For this review, use the dimensioned drawing (mm, ordinates from the lowest corner) and the shaded views. Coordinates: 2 decimals unless noted, no trailing zeros. Write each loop counter-clockwise with the first axis right and the second up, starting at its lowest first coordinate (ties: lowest second). Pieces come first, ordered by that corner, then holes. Notation, with made-up numbers: (86.25, 60.5) - (117.25, 60.5) arc R27 cw to (117.25, 97.5) - close; hole circle Ø4 at (6, 33). An arc over 180 degrees is marked (long way). Put each result on its own line as item: value.
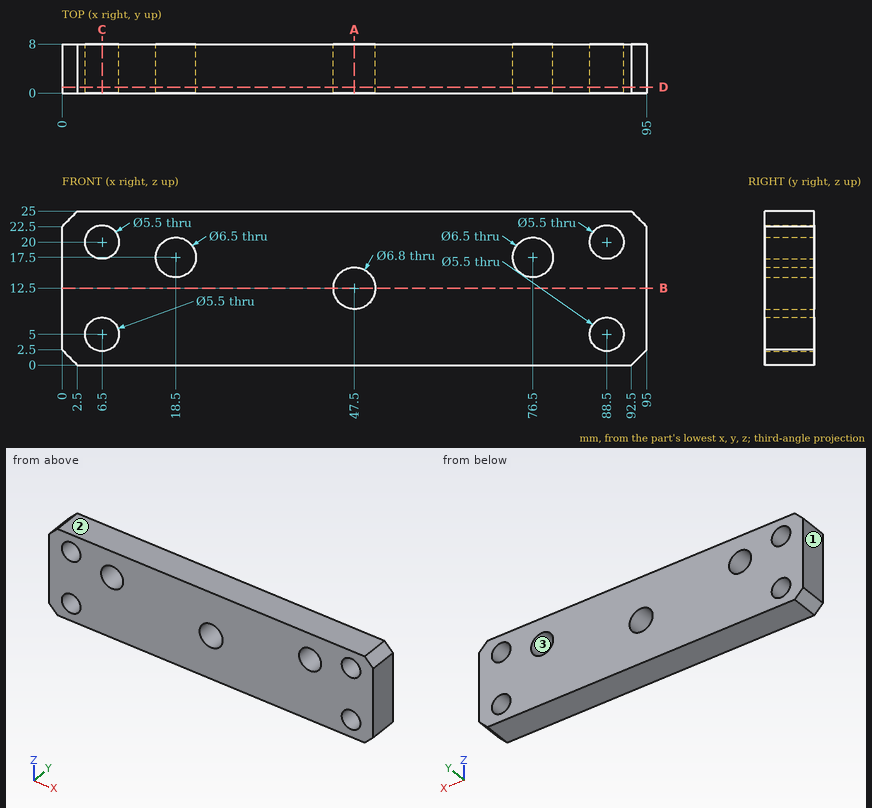
1. Consider section B-B on z = 12.5. State the section outline as (x, y) points, plus the area to 3 significant figures.
Determined:
outline: (0, 0) - (44.1, 0) - (44.1, 8) - (0, 8) - close; (50.9, 0) - (95, 0) - (95, 8) - (50.9, 8) - close
area: 706 mm^2
2. Consider section A-A on x = 47.5. State the section outline as (y, z) points, plus the area to 3 significant figures.
Determined:
outline: (0, 0) - (8, 0) - (8, 9.1) - (0, 9.1) - close; (0, 15.9) - (8, 15.9) - (8, 25) - (0, 25) - close
area: 146 mm^2
3. Consider section C-C on x = 6.5. State the section outline as (y, z) points.
Determined:
outline: (0, 0) - (8, 0) - (8, 2.25) - (0, 2.25) - close; (0, 7.75) - (8, 7.75) - (8, 17.25) - (0, 17.25) - close; (0, 22.75) - (8, 22.75) - (8, 25) - (0, 25) - close
4. To check wall thickness, follow probe 1 along X at (y, z) = (7, 4.75); probe 2 along Z at (x, y) = (6.5, 2.25); probe 3 along Z at (x, y) = (76.5, 5.75). State the ranges of each line that lie inside material, in increasing order.
Determined:
probe 1: x = 0 to 3.76, 9.24 to 85.76, 91.24 to 95
probe 2: z = 0 to 2.25, 7.75 to 17.25, 22.75 to 25
probe 3: z = 0 to 14.25, 20.75 to 25
5. Consider section D-D on y = 1. State the section outline as (x, z) points, plus the area to 3 significant figures.
Determined:
outline: (0, 2.5) - (2.5, 0) - (92.5, 0) - (95, 2.5) - (95, 22.5) - (92.5, 25) - (2.5, 25) - (0, 22.5) - close; hole circle Ø5.5 at (6.5, 5); hole circle Ø5.5 at (6.5, 20); hole circle Ø6.5 at (18.5, 17.5); hole circle Ø6.8 at (47.5, 12.5); hole circle Ø6.5 at (76.5, 17.5); hole circle Ø5.5 at (88.5, 5); hole circle Ø5.5 at (88.5, 20)
area: 2,160 mm^2
6. The part is to be moulded in two halves that separate along X. For the marked faces 1, 2 and 3, say which applies: +X half, -X half, draft (parallel to the pull), parting line (faces both ways), or undercut.
Determined:
face 1: -X half
face 2: draft
face 3: undercut
